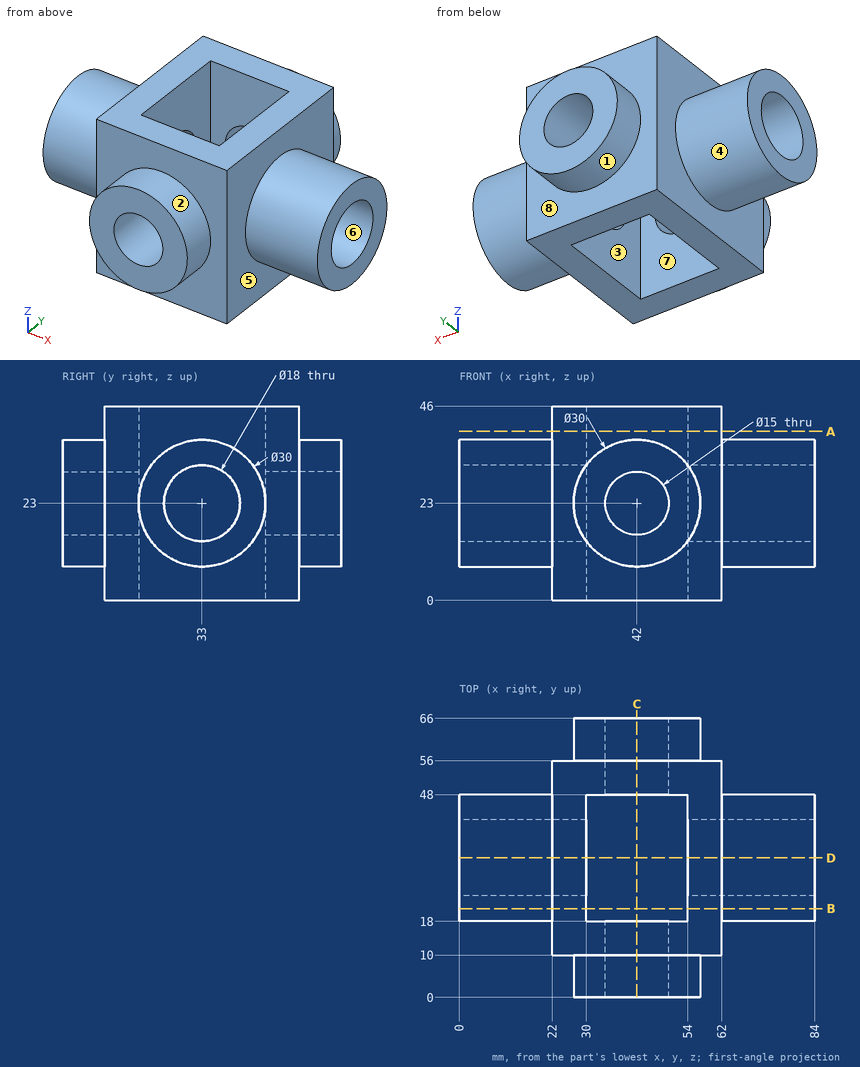
The drawing under review shows one solid part. Ordinate dimensions are in mm from its lowest x, y, z. A direction names the side the tool comes from. Round coordinates to 2 decimals unless told otherwise and drop trailing zeros. Write each loop counter-clockwise with the first axis right and the second up, starting at its lowest first coordinate (ties: lowest second). Pieces come first, ordered by that corner, then holes. Notation, with made-up numbers: (73, -1.75) -> (78, -1.75) arc R15 ccw to (78, 6.25) -> close; hole circle Ø4 at (34.25, 79.5). An arc over 180 degrees is marked (long way). Put each result on its own line as item: value.
Q1. Consider section B-B on y = 21. State the section outline as (x, z) points, and give its area (3 significant figures).
Determined:
outline: (0, 14) -> (22, 14) -> (22, 0) -> (30, 0) -> (30, 46) -> (22, 46) -> (22, 32) -> (0, 32) -> close; (54, 0) -> (62, 0) -> (62, 14) -> (84, 14) -> (84, 32) -> (62, 32) -> (62, 46) -> (54, 46) -> close
area: 1,530 mm^2
Q2. Machinability: for the marked faces 1, 2, 3 and 4, which of the approach directions +Z, -Z, +X, -X, +Y, -Y give a long, thin tool a straight path to every point of the face, cutting with its end or side? Answer none if there is none.
Determined:
face 1: +Y
face 2: -Y
face 3: +Z, -Z
face 4: -X
Q3. The part is to be moulded in two halves that separate along Y. For the marked faces 5, 6, 7 and 8, say which applies: released by +Y, released by -Y, zero draft, split by the parting line, or undercut.
Determined:
face 5: zero draft
face 6: undercut
face 7: undercut
face 8: released by +Y
Q4. Consider section D-D on y = 33. State the section outline as (x, z) points.
Determined:
outline: (0, 8) -> (22, 8) -> (22, 0) -> (30, 0) -> (30, 14) -> (0, 14) -> close; (0, 32) -> (30, 32) -> (30, 46) -> (22, 46) -> (22, 38) -> (0, 38) -> close; (54, 0) -> (62, 0) -> (62, 8) -> (84, 8) -> (84, 14) -> (54, 14) -> close; (54, 32) -> (84, 32) -> (84, 38) -> (62, 38) -> (62, 46) -> (54, 46) -> close
Q5. Clearance check with a flat-ended pin moving along its axis: pin 1 Ø5 at (y, z) = (28.5, 40.5) entering from -X. State where the tip first meets the part, or that it passes through.
Determined:
pin 1: stops at x = 22
Q6. Consider section A-A on z = 40. State the section outline as (x, y) points, and give its area (3 significant figures).
Determined:
outline: (22, 10) -> (62, 10) -> (62, 56) -> (22, 56) -> close; hole (30, 18) -> (54, 18) -> (54, 48) -> (30, 48) -> close
area: 1,120 mm^2
Q7. Consider section C-C on x = 42. State the section outline as (y, z) points, and give its area (3 significant figures).
Determined:
outline: (0, 8) -> (10, 8) -> (10, 0) -> (18, 0) -> (18, 15.5) -> (0, 15.5) -> close; (0, 30.5) -> (18, 30.5) -> (18, 46) -> (10, 46) -> (10, 38) -> (0, 38) -> close; (48, 0) -> (56, 0) -> (56, 8) -> (66, 8) -> (66, 15.5) -> (48, 15.5) -> close; (48, 30.5) -> (66, 30.5) -> (66, 38) -> (56, 38) -> (56, 46) -> (48, 46) -> close
area: 796 mm^2
Q8. To check wall thickness, follow L1, parallel to X at y = 19.5, z = 29; L2, parallel to Z at x = 41.5, y = 14; L3, parallel to X at y = 35, z = 3. State the ranges of each line that lie inside material, in increasing order. Write a range as [from, to].
Determined:
L1: x = [0, 30], [54, 84]
L2: z = [0, 15.52], [30.48, 46]
L3: x = [22, 30], [54, 62]
